Could you check a few things on this model? Use its own coordinates, in mm. Round coordinates to 2 decimals unless told otherwise and drop trailing zeros. Loops run counter-clockwise (first coordinate to the right, second up) from the corner with the lowest first, then second, coordinate; pieces in that order, holes last. Notation, with made-up numbers: M -24.75,-9 L 9.25,-9 A28 ccw 9.25,15 Z; hole C 49.5,87.25 d6. An arc over 180 degrees is marked long. Answer in a Markdown table with one row per item.
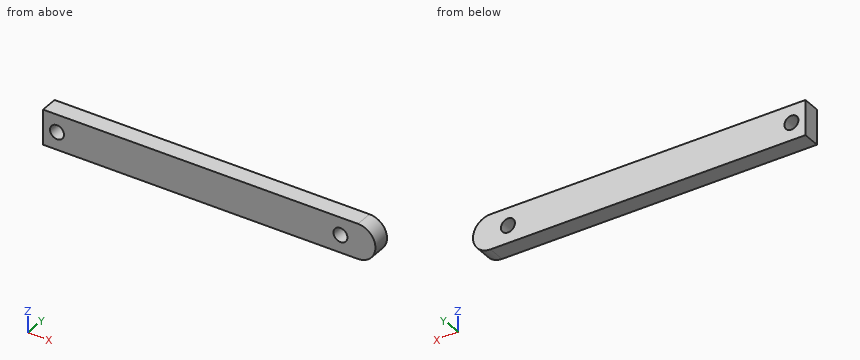
```python
from build123d import *

# Parameters (mm, degrees)
SKETCH1_R           = 2
BOSS_EXTRUDE1_DEPTH = 5


with BuildPart() as part:
    # Sketch1 → Boss-Extrude1 (new body)
    with BuildSketch(Plane(origin=(0, 0, 0), x_dir=(1, 0, 0), z_dir=(0, 1, 0))):
        with BuildLine():
            Line((0, 5), (0, 0))
            Line((0, 0), (90, 0))
            ThreePointArc((90, 0), (95, 5), (90, 10))
            Line((90, 10), (0, 10))
            Line((0, 10), (0, 5))
        make_face()
        with Locations(Location((4, 5, 0), (0, 0, 270))):
            Circle(SKETCH1_R, mode=Mode.SUBTRACT)
        with Locations(Location((85, 5, 0), (0, 0, 270))):
            Circle(SKETCH1_R, mode=Mode.SUBTRACT)
    extrude(amount=BOSS_EXTRUDE1_DEPTH)


solid = part.part
```
1) I want a section at B-B, the plane y = 3.5. Please give me the cut outline in (x, z), plus the area to 3 significant figures.
Computed:
| item | result |
|---|---|
| outline | M 0,-10 L 90,-10 A5 ccw 90,0 L 0,0 Z; hole C 4,-5 d4; hole C 85,-5 d4 |
| area | 914 mm² |
2) I want a section at A-A, the plane z = -5. Please give me the cut outline in (x, y).
Computed:
| item | result |
|---|---|
| outline | M 0,0 L 2,0 L 2,5 L 0,5 Z; M 6,0 L 83,0 L 83,5 L 6,5 Z; M 87,0 L 95,0 L 95,5 L 87,5 Z |
3) Will this pin go through, and if not, where does the flat tip stop? P1, Ø3.5, axis at x = 85, z = -5, coming from the -Y side.
Computed:
| item | result |
|---|---|
| P1 | passes through |
4) I need wall thicknesses on line 1 (X direction, y = 3.15, z = -5); line 2 (X direction, y = 1.5, z = -4.5); line 3 (Z direction, x = 84, y = 3.4). Which ranges of each line are inside material? Lowest first, please.
Computed:
| item | result |
|---|---|
| line 1 | x = 0 to 2, 6 to 83, 87 to 95 |
| line 2 | x = 0 to 2.06, 5.94 to 83.06, 86.94 to 94.97 |
| line 3 | z = -10 to -6.73, -3.27 to 0 |
5) I want a section at C-C, the plane x = 85. Please give me the cut outline in (y, z).
Computed:
| item | result |
|---|---|
| outline | M 0,-10 L 5,-10 L 5,-7 L 0,-7 Z; M 0,-3 L 5,-3 L 5,0 L 0,0 Z |
